Geometry: final body of the model. Coordinates: model frame, mm. A direction names the side the tool comes from. Give positions to 0.01 mm unless a question says otherwise; leave off trailing zeros. Write each loop counter-clockwise with the first axis right and the second up, starting at its lowest first coordinate (ties: lowest second). Pieces come first, ordered by that corner, then holes.
```python
from build123d import *

# Parameters (mm, degrees)
BOSS_EXTRUDE1_DEPTH = 152
SKETCH3_R           = 10
BOSS_EXTRUDE2_DEPTH = 2.5
BOSS_EXTRUDE3_DEPTH = 2.5


with BuildPart() as part:
    # Sketch1 → Revolve1 (revolve)
    with BuildSketch(Plane.XY):
        Polygon((0, 0), (4.875, 0), (4.875, 3), (4.225, 3), (4.225, 5), (6.5, 5), (6.5, 6), (0, 6), align=None)
    revolve(axis=Axis((0, 6, 0), (0, -1, 0)))

    # Sketch2 → Boss-Extrude1 (add)
    with BuildSketch(Plane(origin=(0, 6, 0), x_dir=(1, 0, 0), z_dir=(0, 1, 0))):
        with BuildLine():
            Line((-1, 4.5), (-1, 1.5))
            ThreePointArc((-1, 1.5), (-1.146446609, 1.146446609), (-1.5, 1))
            Line((-1.5, 1), (-4.5, 1))
            ThreePointArc((-4.5, 1), (-5.5, 0), (-4.5, -1))
            Line((-4.5, -1), (-1.5, -1))
            ThreePointArc((-1.5, -1), (-1.146446609, -1.146446609), (-1, -1.5))
            Line((-1, -1.5), (-1, -4.5))
            ThreePointArc((-1, -4.5), (0, -5.5), (1, -4.5))
            Line((1, -4.5), (1, -1.5))
            ThreePointArc((1, -1.5), (1.146446609, -1.146446609), (1.5, -1))
            Line((1.5, -1), (4.5, -1))
            ThreePointArc((4.5, -1), (5.5, 0), (4.5, 1))
            Line((4.5, 1), (1.5, 1))
            ThreePointArc((1.5, 1), (1.146446609, 1.146446609), (1, 1.5))
            Line((1, 1.5), (1, 4.5))
            ThreePointArc((1, 4.5), (0, 5.5), (-1, 4.5))
        make_face()
    extrude(amount=BOSS_EXTRUDE1_DEPTH)

    # Sketch3 → Boss-Extrude2 (add)
    with BuildSketch(Plane(origin=(0, 158, 0), x_dir=(1, 0, 0), z_dir=(0, 1, 0))):
        Circle(SKETCH3_R)
    extrude(amount=BOSS_EXTRUDE2_DEPTH)

    # Sketch4 → Boss-Extrude3 (add)
    with BuildSketch(Plane(origin=(0, 160.5, 0), x_dir=(1, 0, 0), z_dir=(0, 1, 0))):
        with BuildLine():
            ThreePointArc((1, 8), (0, 9), (-1, 8))
            Line((-1, 8), (-1, -8))
            ThreePointArc((-1, -8), (0, -9), (1, -8))
            Line((1, -8), (1, 8))
        make_face()
        with BuildLine():
            ThreePointArc((-2.5, 6), (-3.5, 7), (-4.5, 6))
            Line((-4.5, 6), (-4.5, -6))
            ThreePointArc((-4.5, -6), (-3.5, -7), (-2.5, -6))
            Line((-2.5, -6), (-2.5, 6))
        make_face()
        with BuildLine():
            ThreePointArc((4.5, 6), (3.5, 7), (2.5, 6))
            Line((2.5, 6), (2.5, -6))
            ThreePointArc((2.5, -6), (3.5, -7), (4.5, -6))
            Line((4.5, -6), (4.5, 6))
        make_face()
        with BuildLine():
            ThreePointArc((6, 4), (7, 5), (8, 4))
            Line((8, 4), (8, -4))
            ThreePointArc((8, -4), (7, -5), (6, -4))
            Line((6, -4), (6, 4))
        make_face()
        with BuildLine():
            Line((-6, -4), (-6, 4))
            ThreePointArc((-6, 4), (-7, 5), (-8, 4))
            Line((-8, 4), (-8, -4))
            ThreePointArc((-8, -4), (-7, -5), (-6, -4))
        make_face()
    extrude(amount=BOSS_EXTRUDE3_DEPTH)


solid = part.part
```
Item 1: Pull-direction query (X, two-part tool) for faces 5 (the face through (-2.5, 162, 0)), 6 (the face through (0, 0, 0)), 7 (the face through (8, 162, 0)); classes: +X half, -X half, draft (parallel to the pull), parting line (faces both ways), or undercut.
Found:
face 5: undercut
face 6: draft
face 7: +X half
Item 2: Pin query (flat end, axial travel): pin 1 Ø1.5 at (x, y) = (-3, 105) entering from -Z; pin 2 Ø1.2 at (y, z) = (161.5, 0) entering from -X; pin 3 Ø5 at (y, z) = (131.5, -4) entering from -X. Return the tip coordinate at first contact, or that it passes through.
Found:
pin 1: stops at z = -1
pin 2: stops at x = -8
pin 3: stops at x = -1
Item 3: Line query: L1, parallel to Y at x = 4, z = -1.5; L2, parallel to Y at x = 2, z = 2.75; L3, parallel to Y at x = -3.25, z = 2.5. Output: solid intervals per line, ascending.
Found:
L1: y = 0 to 3, 5 to 6, 158 to 163
L2: y = 0 to 6, 158 to 160.5
L3: y = 0 to 6, 158 to 163
Item 4: Reachability of faces 1 (the face through (-4, 3, 2)), 2 (the face through (3, 81, -1)), 3 (the face through (-1, 81, -3)), 4 (the face through (-6, 162, 0)) from +Z, -Z, +X, -X, +Y, -Y: full face, straight path, thin tool, end or side. Return the list, or none.
Found:
face 1: none
face 2: -Z, +X
face 3: -Z, -X
face 4: +Z, -Z, +Y
Item 5: Section A-A, the plane y = 93. Return the cut outline in (x, z).
Found:
outline: (-4.5, -1) - (-1.5, -1) arc R0.5 cw to (-1, -1.5) - (-1, -4.5) arc R1 ccw to (1, -4.5) - (1, -1.5) arc R0.5 cw to (1.5, -1) - (4.5, -1) arc R1 ccw to (4.5, 1) - (1.5, 1) arc R0.5 cw to (1, 1.5) - (1, 4.5) arc R1 ccw to (-1, 4.5) - (-1, 1.5) arc R0.5 cw to (-1.5, 1) - (-4.5, 1) arc R1 ccw to start
